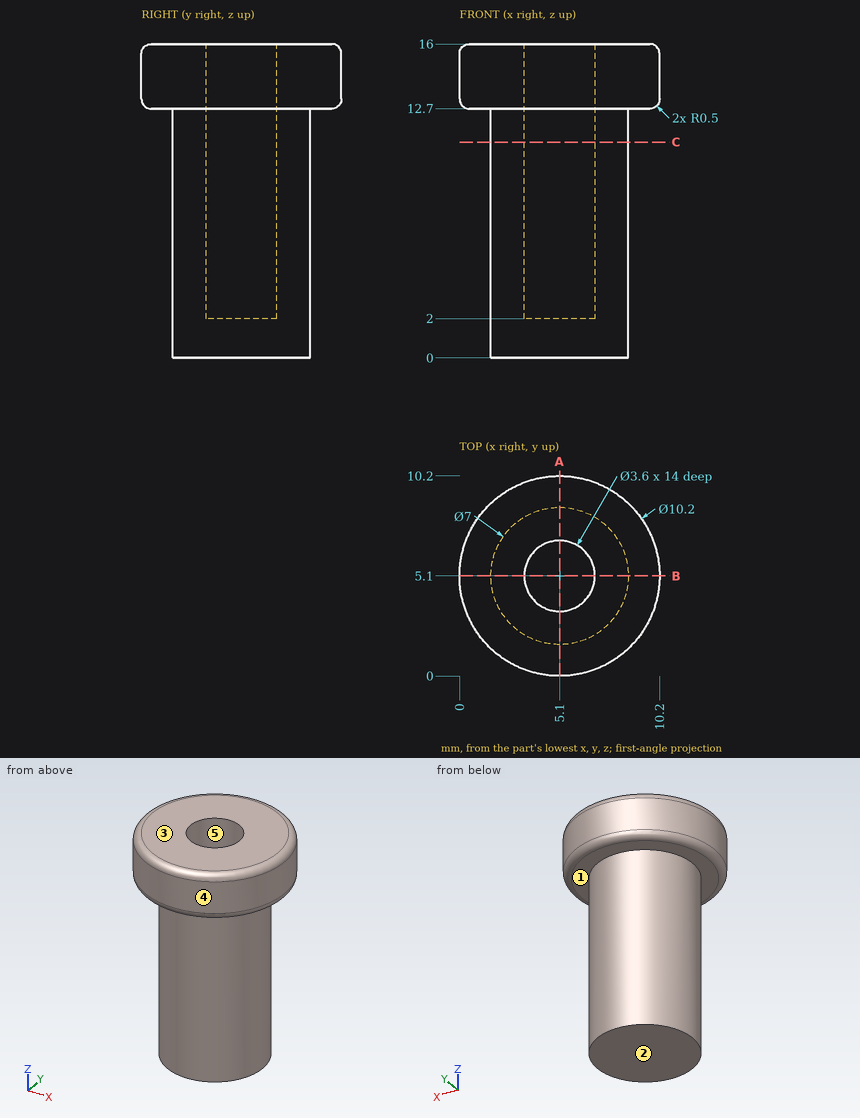
Check sheet for the drawn part. Datum: minimum x, y, z corner. Units: mm. A direction names the side the tool comes from. Round coordinates to 2 decimals unless told otherwise and drop trailing zeros. Write each loop counter-clockwise with the first axis right and the second up, starting at its lowest first coordinate (ties: lowest second). Pieces come first, ordered by that corner, then holes. Notation, with made-up numbers: (24.25, 44.25) -> (68.25, 44.25) arc R24 cw to (68.25, 65.25) -> close; hole circle Ø9 at (-21.5, 70). An arc over 180 degrees is marked (long way). Write each question's results on one line, items separated by ' | '.
Q1. Sectioned sample at A-A, the plane x = 5.1. Record the boundary of the cut face in (y, z), and give its area (3 significant figures).
Derived:
outline: (0, 13.2) arc R0.5 ccw to (0.5, 12.7) -> (1.6, 12.7) -> (1.6, 0) -> (8.6, 0) -> (8.6, 12.7) -> (9.7, 12.7) arc R0.5 ccw to (10.2, 13.2) -> (10.2, 15.5) arc R0.5 ccw to (9.7, 16) -> (6.9, 16) -> (6.9, 2) -> (3.3, 2) -> (3.3, 16) -> (0.5, 16) arc R0.5 ccw to (0, 15.5) -> close | area: 71.9 mm²
Q2. Draft check along Y on the marked faces 3, 4 and 5. Enter one of: released by +Y, released by -Y, zero draft, split by the parting line, or undercut.
Derived:
face 3: zero draft | face 4: split by the parting line | face 5: undercut
Q3. Go/stop test with flat-tipped pins: pin 1 Ø3 at (x, z) = (3, 3) entering from -Y; pin 2 Ø1.5 at (x, z) = (4.5, 10.5) entering from +Y; pin 3 Ø1 at (y, z) = (1.5, 4) entering from +X. Record where each tip stops, or that it passes through.
Derived:
pin 1: stops at y = 1.65 | pin 2: stops at y = 8.6 | pin 3: stops at x = 6.72
Q4. Access from +Z, -Z, +X, -X, +Y, -Y to the whole of each face (thin tool, end or side, straight path). Record for the marked faces 1 and 2.
Derived:
face 1: -Z | face 2: -Z, +X, -X, +Y, -Y
Q5. Sectioned sample at C-C, the plane z = 11. Record the boundary of the cut face in (x, y), and give its area (3 significant figures).
Derived:
outline: circle Ø7 at (5.1, 5.1); hole circle Ø3.6 at (5.1, 5.1) | area: 28.3 mm²
Q6. Thickness scan on probe 1 along Y at (x, z) = (5.5, 13) (3 decimals); probe 2 along X at (y, z) = (4.25, 10.75); probe 3 along Z at (x, y) = (4, 8.5). Record the ranges inside material, lowest first.
Derived:
probe 1: y = 0.058 to 3.345, 6.855 to 10.142 | probe 2: x = 1.7 to 3.51, 6.69 to 8.5 | probe 3: z = 12.7 to 16
